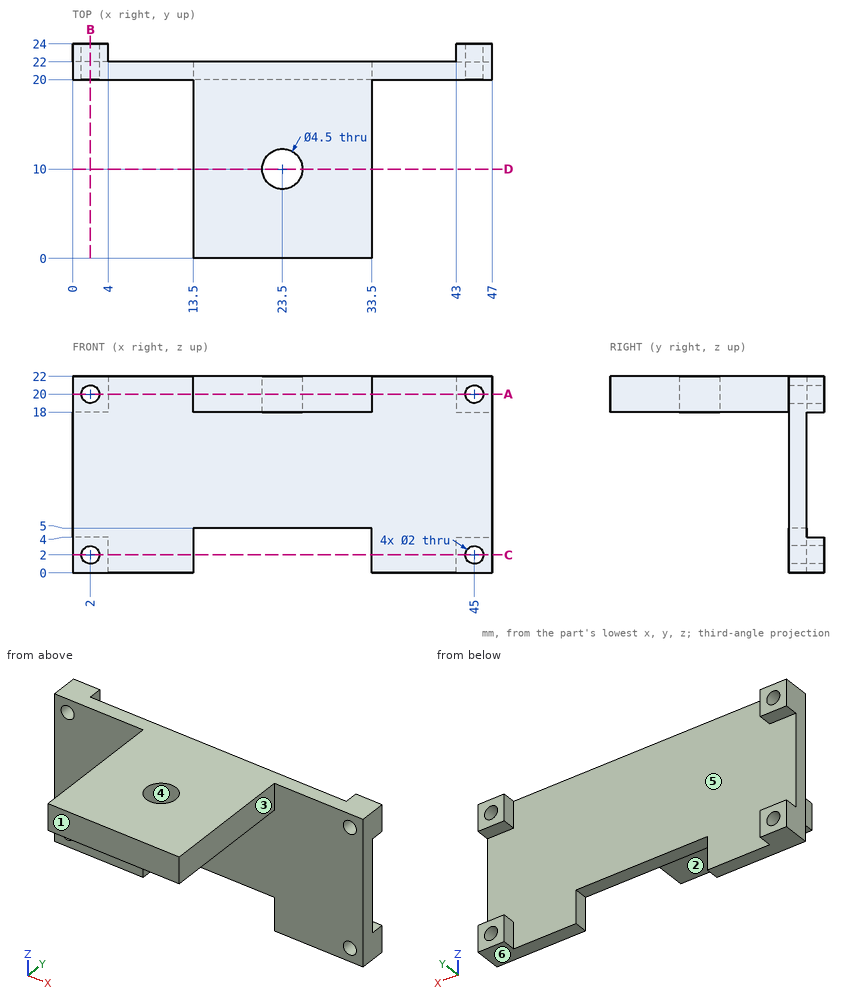
Study the drawing (mm; zero at the part's minimum x, y, z) and answer. A direction names the side the tool comes from. Give positions to 0.01 mm unless a question says otherwise; leave off trailing zeros. Order: outer loops, then holes, each group sorted by start corner. A loop starts at its lowest first (then second) coordinate and runs counter-clockwise, first axis right, second up. Notation, with made-up numbers: (27.25, 80.5) - (76.25, 80.5) arc R27 cw to (76.25, 116.5) - close; hole circle Ø10 at (6, 25.5). An arc over 180 degrees is marked (long way). Answer as CSV lines item,"result". Start each with the question number.
Q1. Given pin 1 Ø1.2 at (y, z) = (8, 21) entering from -X; pin 2 Ø1.8 at (x, z) = (2, 20) entering from -Y (3 decimals); pin 3 Ø1.5 at (x, z) = (6.5, 18.5) entering from +Y; pin 4 Ø5 at (x, y) = (33, 16.5) entering from -Z, each flat-ended and moving along its own axis, determine where each tip first touches the part or whether it passes through.
Q2. Find the intervals of material crossed by L1, parallel to X at y = 21.95, z = 20; L2, parallel to Z at x = 2, y = 23; L3, parallel to X at y = 22.4, z = 2, in increasing order. Write a range as [from, to].
Q3. For the marked faces 1 and 2, determine the directions among +Z, -Z, +X, -X, +Y, -Y from which every point of the face is accessible in a straight line to the end or side of a thin tool.
Q4. The part is cut by section C-C (z = 2). Write down the section's boundary in (x, y).
Q5. The part is cut by section D-D (y = 10). Write down the section's boundary in (x, z).
Q6. The part is cut by section A-A (z = 20). Write down the section's boundary in (x, y).
Q7. The part is cut by section B-B (x = 2). Write down the section's boundary in (y, z), then the cut area to 3 significant figures.
Q8. The mould has two halves that part along X. Classify the marked faces 3, 4, 5 and 6: +X half, -X half, draft (parallel to the pull), parting line (faces both ways), or undercut.
Check result:
1,pin 1,"stops at x = 13.5"
1,pin 2,"passes through"
1,pin 3,"stops at y = 22"
1,pin 4,"stops at z = 18"
2,L1,"x = [0, 1], [3, 44], [46, 47]"
2,L2,"z = [0, 1], [3, 4], [18, 19], [21, 22]"
2,L3,"x = [0, 1], [3, 4], [43, 44], [46, 47]"
3,face 1,"+Z, -Z, +X, -X, -Y"
3,face 2,"-Z, +X, -X, -Y"
4,outline,"(0, 20) - (1, 20) - (1, 24) - (0, 24) - close; (3, 20) - (13.5, 20) - (13.5, 22) - (4, 22) - (4, 24) - (3, 24) - close; (33.5, 20) - (44, 20) - (44, 24) - (43, 24) - (43, 22) - (33.5, 22) - close; (46, 20) - (47, 20) - (47, 24) - (46, 24) - close"
5,outline,"(13.5, 18) - (21.25, 18) - (21.25, 22) - (13.5, 22) - close; (25.75, 18) - (33.5, 18) - (33.5, 22) - (25.75, 22) - close"
6,outline,"(0, 20) - (1, 20) - (1, 24) - (0, 24) - close; (3, 20) - (13.5, 20) - (13.5, 0) - (33.5, 0) - (33.5, 20) - (44, 20) - (44, 24) - (43, 24) - (43, 22) - (4, 22) - (4, 24) - (3, 24) - close; (46, 20) - (47, 20) - (47, 24) - (46, 24) - close; hole circle Ø4.5 at (23.5, 10)"
7,outline,"(20, 0) - (24, 0) - (24, 1) - (20, 1) - close; (20, 3) - (24, 3) - (24, 4) - (22, 4) - (22, 18) - (24, 18) - (24, 19) - (20, 19) - close; (20, 21) - (24, 21) - (24, 22) - (20, 22) - close"
7,area,"44.0 mm²"
8,face 3,"+X half"
8,face 4,"undercut"
8,face 5,"undercut"
8,face 6,"draft"
